Read the model definition and answer for the solid it produces. Units are mm, in the model's axes. Coordinates: 2 decimals unless noted, no trailing zeros. Write each loop counter-clockwise with the first axis right and the second up, starting at its lowest first coordinate (ties: lowest second). Pieces come first, ordered by that corner, then holes.
1) Determine the mould class of faces 1 (the face through (0, 4, 0)), 2 (the face through (22.854, -10.676, 2.535)), 3 (the face through (0, -15, 2)) for opening direction Y: +Y half, -Y half, draft (parallel to the pull), parting line (faces both ways), or undercut.
2) Find the intervals of material crossed by line 1 (X direction, y = -10, z = 4.5); line 2 (Y direction, x = -25, z = 3.5); line 3 (X direction, y = -12, z = 2.7), in increasing order.
3) The part is cut by section C-C (z = 3.1). Determine the outline of the cut face in (x, y), then the cut area to 3 significant figures.
4) The part is cut by section B-B (y = -1.5). Determine the outline of the cut face in (x, z), then the cut area to 3 significant figures.
5) The part is cut by section D-D (x = 0). Determine the outline of the cut face in (y, z).
6) The part is cut by section A-A (x = 25). Determine the outline of the cut face in (y, z), then the cut area to 3 significant figures.
7) This flat-tipped pin is pushed along its axis until it touches: pin 1 Ø6 at (x, y) = (-25, 10) entering from -Z. Where does it stop, or does it pass through?
from build123d import *

# Parameters (mm, degrees)
F0_W     = 60
F0_H     = 30
F0_R     = 2.3276223463
F0_R_2   = 2.3015247155
F0_R_3   = 2.1862089509
F0_R_4   = 12
F0_R_5   = 1.5601782255
F1_DEPTH = 5
F2_D     = 4.5
F3_D     = 5.5


with BuildPart() as f1:
    # F0 (on Top) → F1 (new body)
    with BuildSketch(Plane.XY):
        Rectangle(F0_W, F0_H)
        with Locations((-25, -10)):
            Circle(F0_R, mode=Mode.SUBTRACT)
        with Locations((25, -10)):
            Circle(F0_R_2, mode=Mode.SUBTRACT)
        with Locations((-25, 10)):
            Circle(F0_R_3, mode=Mode.SUBTRACT)
        Circle(F0_R_4, mode=Mode.SUBTRACT)
        with Locations((25, 10)):
            Circle(F0_R_5, mode=Mode.SUBTRACT)
        Circle(F0_R_4)
        with BuildLine():
            ThreePointArc((-2.5620431112, -6.5142869983), (0.0664242114, 6.9996848375), (2.4379568888, -6.5617349999))
            Line((2.4379568888, -6.5617349999), (2.4379568888, -9.5))
            Line((2.4379568888, -9.5), (-2.5620431112, -9.5))
            Line((-2.5620431112, -9.5), (-2.5620431112, -6.5142869983))
        make_face(mode=Mode.SUBTRACT)
        with BuildLine():
            Line((2.4379568888, -9.5), (2.4379568888, -6.5617349999))
            ThreePointArc((2.4379568888, -6.5617349999), (0.0664242114, 6.9996848375), (-2.5620431112, -6.5142869983))
            Line((-2.5620431112, -6.5142869983), (-2.5620431112, -9.5))
            Line((-2.5620431112, -9.5), (2.4379568888, -9.5))
        make_face()
        with Locations((-25, -10)):
            Circle(F0_R)
        with Locations((25, -10)):
            Circle(F0_R_2)
        with Locations((-25, 10)):
            Circle(F0_R_3)
        with Locations((25, 10)):
            Circle(F0_R_5)
    extrude(amount=F1_DEPTH)

    # F2 (through all)
    with Locations(Plane(origin=(0, 0, 0), x_dir=(1, 0, 0), z_dir=(0, 0, -1))):
        with Locations((25, -10), (-25, -10), (-25, 10), (25, 10)):
            Hole(F2_D / 2)

    # F3 (through all)
    with Locations(Plane(origin=(0, 0, 0), x_dir=(1, 0, 0), z_dir=(0, 0, -1))):
        with Locations((0, 0)):
            Hole(F3_D / 2)


solid = f1.part
Reported:
1. face 1: draft
1. face 2: undercut
1. face 3: -Y half
2. line 1: x = -30 to -27.25, -22.75 to 22.75, 27.25 to 30
2. line 2: y = -15 to -12.25, -7.75 to 7.75, 12.25 to 15
2. line 3: x = -30 to -26.03, -23.97 to 23.97, 26.03 to 30
3. outline: (-30, -15) - (30, -15) - (30, 15) - (-30, 15) - close; hole circle Ø4.5 at (-25, -10); hole circle Ø4.5 at (-25, 10); hole circle Ø5.5 at (0, 0); hole circle Ø4.5 at (25, -10); hole circle Ø4.5 at (25, 10)
3. area: 1,710 mm2
4. outline: (-30, 0) - (-2.3, 0) - (-2.3, 5) - (-30, 5) - close; (2.3, 0) - (30, 0) - (30, 5) - (2.3, 5) - close
4. area: 277 mm2
5. outline: (-15, 0) - (-2.75, 0) - (-2.75, 5) - (-15, 5) - close; (2.75, 0) - (15, 0) - (15, 5) - (2.75, 5) - close
6. outline: (-15, 0) - (-12.25, 0) - (-12.25, 5) - (-15, 5) - close; (-7.75, 0) - (7.75, 0) - (7.75, 5) - (-7.75, 5) - close; (12.25, 0) - (15, 0) - (15, 5) - (12.25, 5) - close
6. area: 105 mm2
7. pin 1: stops at z = 0
